Input: part model. Units: mm. Frame: model coordinates. Round coordinates to 2 decimals unless told otherwise and drop trailing zeros. Loops run counter-clockwise (first coordinate to the right, second up) from the corner with the lowest first, then second, coordinate; pieces in that order, holes last.
(1) First-contact query: pin 1 Ø11.5 at (x, y) = (188, 0) entering from -Z; pin 2 Ø3 at (x, z) = (25, 1.5) entering from -Y. Flat tips, straight axial feed; report the tip coordinate or a pass-through.
(2) Cut plane A-A, the plane z = -1.5. Output: boundary loops of the cut face in (x, y).
(3) Cut plane B-B, the plane y = 0. Output: boundary loops of the cut face in (x, z).
(4) Line query: line 1 (Y direction, x = 188, z = -0.95); line 2 (Y direction, x = 18, z = 0.9); line 3 (Y direction, x = 161.5, z = 1.85). Output: solid intervals per line, ascending.
(5) Cut plane C-C, the plane x = 94. Output: boundary loops of the cut face in (y, z).
(6) Cut plane D-D, the plane x = 62.5. Output: boundary loops of the cut face in (y, z).
from build123d import *

# Parameters (mm, degrees)
SKETCH1_R           = 5
BOSS_EXTRUDE1_DEPTH = 3
FILLET1_R           = 50


with BuildPart() as part:
    # Sketch1 → Boss-Extrude1 (new, symmetric)
    with BuildSketch(Plane.XY):
        with BuildLine():
            Line((2, 24.919871589), (2, 19.919871589))
            Line((2, 19.919871589), (-2, 19.919871589))
            Line((-2, 19.919871589), (-2, 24.919871589))
            Line((-2, 24.919871589), (-2, 39.919871589))
            Line((-2, 39.919871589), (17, 39.919871589))
            Line((17, 39.919871589), (60.16248371, 15))
            Line((60.16248371, 15), (188, 15))
            ThreePointArc((188, 15), (203, 0), (188, -15))
            Line((188, -15), (60.16248371, -15))
            Line((60.16248371, -15), (17, -39.919871589))
            Line((17, -39.919871589), (-2, -39.919871589))
            Line((-2, -39.919871589), (-2, -24.919871589))
            Line((-2, -24.919871589), (-2, -19.919871589))
            Line((-2, -19.919871589), (2, -19.919871589))
            Line((2, -19.919871589), (2, -24.919871589))
            ThreePointArc((2, -24.919871589), (12.5, -21.650635095), (20.581241855, -14.191986602))
            Line((20.581241855, -14.191986602), (16.251114836, -11.691986602))
            Line((16.251114836, -11.691986602), (18.251114836, -8.227884987))
            Line((18.251114836, -8.227884987), (22.581241855, -10.727884987))
            ThreePointArc((22.581241855, -10.727884987), (25, 0), (22.581241855, 10.727884987))
            Line((22.581241855, 10.727884987), (18.251114836, 8.227884987))
            Line((18.251114836, 8.227884987), (16.251114836, 11.691986602))
            Line((16.251114836, 11.691986602), (20.581241855, 14.191986602))
            ThreePointArc((20.581241855, 14.191986602), (12.5, 21.650635095), (2, 24.919871589))
        make_face()
        with Locations((188, 0)):
            Circle(SKETCH1_R, mode=Mode.SUBTRACT)
    extrude(amount=BOSS_EXTRUDE1_DEPTH, both=True)

    # Fillet1
    fillet1_edges = [part.edges().sort_by_distance(p)[0] for p in [
        (60.16248371, -15, 0),
        (60.16248371, 15, 0),
    ]]
    fillet(fillet1_edges, radius=FILLET1_R)


solid = part.part
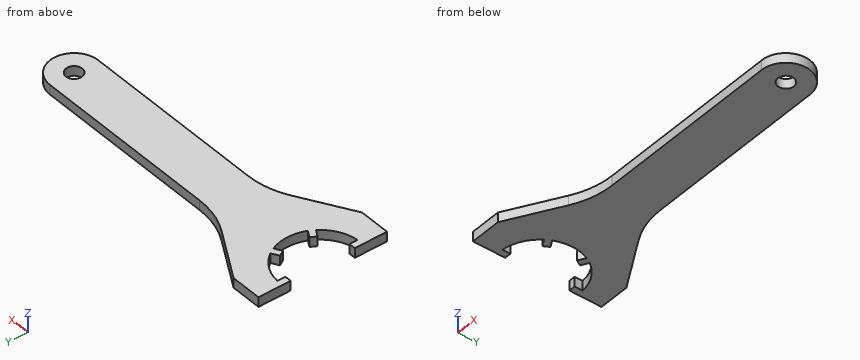
Reported:
1. pin 1: stops at z = -3
1. pin 2: stops at y = -36.17
2. outline: (-2, -39.92) - (17, -39.92) - (48.56, -21.7) arc R50 cw to (73.56, -15) - (188, -15) arc R15 ccw to (188, 15) - (73.56, 15) arc R50 cw to (48.56, 21.7) - (17, 39.92) - (-2, 39.92) - (-2, 19.92) - (2, 19.92) - (2, 24.92) arc R25 cw to (20.58, 14.19) - (16.25, 11.69) - (18.25, 8.23) - (22.58, 10.73) arc R25 cw to (22.58, -10.73) - (18.25, -8.23) - (16.25, -11.69) - (20.58, -14.19) arc R25 cw to (2, -24.92) - (2, -19.92) - (-2, -19.92) - close; hole circle Ø10 at (188, 0)
3. outline: (25, -3) - (183, -3) - (183, 3) - (25, 3) - close; (193, -3) - (203, -3) - (203, 3) - (193, 3) - close
4. line 1: y = -15 to -5, 5 to 15
4. line 2: y = -39.34 to -17.35, -12.7 to -8.66, 8.66 to 12.7, 17.35 to 39.34
4. line 3: y = -15 to 15
5. outline: (-15, -3) - (15, -3) - (15, 3) - (-15, 3) - close
6. outline: (-16.24, -3) - (16.24, -3) - (16.24, 3) - (-16.24, 3) - close
